Read the model definition and answer for the solid it produces. Units are mm, in the model's axes. Coordinates: 2 decimals unless noted, no trailing zeros. Write each loop counter-clockwise with the first axis right and the second up, starting at its lowest first coordinate (ties: lowest second). Pieces come first, ordered by that corner, then holes.
1) Find the intervals of material crossed by line 1 (Y direction, x = 0, z = 5.5); line 2 (Y direction, x = -15, z = 4.5); line 3 (Y direction, x = 14.5, z = 4.75), in increasing order.
2) Each of these flat-tipped pins is pushed along its axis until it touches: pin 1 Ø9 at (x, y) = (0, 64) entering from +Z; pin 2 Ø5 at (x, y) = (-36.5, 62.5) entering from -Z; pin 3 Ø3 at (x, y) = (2.5, -56.5) entering from -Z; pin 4 Ø2.5 at (x, y) = (0, -12) entering from -Z. Where does it stop, or does it pass through?
3) The part is cut by section A-A (y = -26.28). Determine the outline of the cut face in (x, z).
4) The part is cut by section D-D (y = 64). Determine the outline of the cut face in (x, z), then the cut area to 3 significant figures.
5) The part is cut by section B-B (z = 2). Give the number of separate pieces and of enclosed holes in the cut face, then the cut area to 3 significant figures.
6) The part is cut by section C-C (x = 0). Determine the outline of the cut face in (y, z), then the cut area to 3 significant figures.
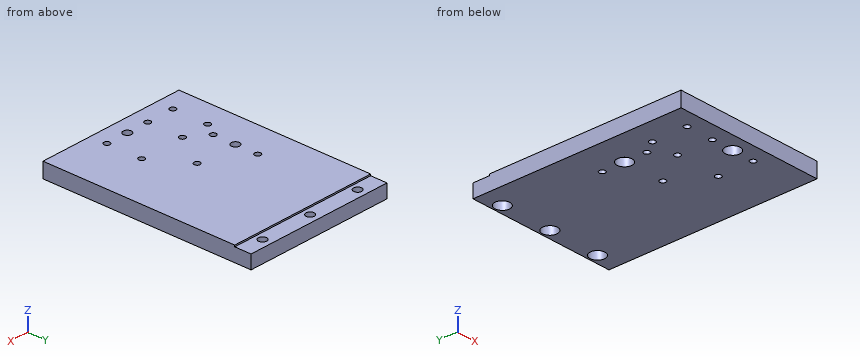
from build123d import *

# Parameters (mm, degrees)
SKIZZE1_W                                            = 100
SKIZZE1_H                                            = 140
AUFSATZ_LINEAR_AUSTRAGEN1_DEPTH                      = 10
STIRNSENKUNG_F_R_M5_ZYLINDERSCHRAUBE_MIT_D           = 5.5
STIRNSENKUNG_F_R_M5_ZYLINDERSCHRAUBE_MIT_CBORE_D     = 10
STIRNSENKUNG_F_R_M5_ZYLINDERSCHRAUBE_MIT_CBORE_DEPTH = 5.4
SKIZZE8_W                                            = 100
SKIZZE8_H                                            = 11
SCHNITT_LINEAR_AUSTRAGEN1_DEPTH                      = 1
STIRNSENKUNG_F_R_M5_ZYLINDERSCHRAUBE_2_D             = 5.5
STIRNSENKUNG_F_R_M5_ZYLINDERSCHRAUBE_2_CBORE_D       = 10
STIRNSENKUNG_F_R_M5_ZYLINDERSCHRAUBE_2_CBORE_DEPTH   = 5.4
F_4_0_4_DURCHMESSER_BOHRUNG1_D                       = 4
F_4_0_4_DURCHMESSER_BOHRUNG2_D                       = 4
F_4_0_4_DURCHMESSER_BOHRUNG3_D                       = 4
F_4_0_4_DURCHMESSER_BOHRUNG4_D                       = 4


with BuildPart() as part:
    # Skizze1 → Aufsatz-Linear austragen1 (new body)
    with BuildSketch(Plane.XY):
        Rectangle(SKIZZE1_W, SKIZZE1_H)
    extrude(amount=AUFSATZ_LINEAR_AUSTRAGEN1_DEPTH)

    # Stirnsenkung f_r M5 Zylinderschraube mit (through all)
    with Locations(Plane(origin=(0, 0, 0), x_dir=(-1, 0, 0), z_dir=(0, 0, -1))):
        with Locations((0, 64), (35, 64), (-35, 64)):
            CounterBoreHole(STIRNSENKUNG_F_R_M5_ZYLINDERSCHRAUBE_MIT_D / 2, STIRNSENKUNG_F_R_M5_ZYLINDERSCHRAUBE_MIT_CBORE_D / 2, STIRNSENKUNG_F_R_M5_ZYLINDERSCHRAUBE_MIT_CBORE_DEPTH)

    # Skizze8 → Schnitt-Linear austragen1 (cut)
    with BuildSketch(Plane.XY.offset(10)):
        with Locations((0, 64.5)):
            Rectangle(SKIZZE8_W, SKIZZE8_H)
    extrude(amount=-SCHNITT_LINEAR_AUSTRAGEN1_DEPTH, mode=Mode.SUBTRACT)

    # Stirnsenkung f_r M5 Zylinderschraube 2 (through all)
    with Locations(Plane(origin=(0, 0, 0), x_dir=(-1, 0, 0), z_dir=(0, 0, -1))):
        with Locations((0, -59), (27.37, -11.28)):
            CounterBoreHole(STIRNSENKUNG_F_R_M5_ZYLINDERSCHRAUBE_2_D / 2, STIRNSENKUNG_F_R_M5_ZYLINDERSCHRAUBE_2_CBORE_D / 2, STIRNSENKUNG_F_R_M5_ZYLINDERSCHRAUBE_2_CBORE_DEPTH)

    # Ø4.0 (4) Durchmesser Bohrung1 (through all)
    with Locations(Plane(origin=(0, 0, 0), x_dir=(-1, 0, 0), z_dir=(0, 0, -1))):
        with Locations((15, -59), (-15, -59), (27.37, -26.28), (27.37, 3.72)):
            Hole(F_4_0_4_DURCHMESSER_BOHRUNG1_D / 2)

    # Ø4.0 (4) Durchmesser Bohrung2 (through all)
    with Locations(Plane(origin=(0, 0, 0), x_dir=(-1, 0, 0), z_dir=(0, 0, -1))):
        with Locations((15, -35.6), (-15, -35.6)):
            Hole(F_4_0_4_DURCHMESSER_BOHRUNG2_D / 2)

    # Ø4.0 (4) Durchmesser Bohrung3 (through all)
    with Locations(Plane.XY.offset(10)):
        with Locations((-33.5, -35.6), (-33.5, -59)):
            Hole(F_4_0_4_DURCHMESSER_BOHRUNG3_D / 2)

    # Ø4.0 (4) Durchmesser Bohrung4 (through all)
    with Locations(Plane.XY.offset(10)):
        with Locations((0, -12)):
            Hole(F_4_0_4_DURCHMESSER_BOHRUNG4_D / 2)


solid = part.part
Reported:
1. line 1: y = -70 to -61.75, -56.25 to -14, -10 to 61.25, 66.75 to 70
1. line 2: y = -70 to -61, -57 to -37.6, -33.6 to 70
1. line 3: y = -70 to -60.94, -57.06 to -37.54, -33.66 to 70
2. pin 1: stops at z = 9
2. pin 2: stops at z = 5.4
2. pin 3: stops at z = 0
2. pin 4: passes through
3. outline: (-50, 0) - (-29.37, 0) - (-29.37, 10) - (-50, 10) - close; (-25.37, 0) - (50, 0) - (50, 10) - (-25.37, 10) - close
4. outline: (-50, 0) - (-40, 0) - (-40, 5.4) - (-37.75, 5.4) - (-37.75, 9) - (-50, 9) - close; (-32.25, 5.4) - (-30, 5.4) - (-30, 0) - (-5, 0) - (-5, 5.4) - (-2.75, 5.4) - (-2.75, 9) - (-32.25, 9) - close; (2.75, 5.4) - (5, 5.4) - (5, 0) - (30, 0) - (30, 5.4) - (32.25, 5.4) - (32.25, 9) - (2.75, 9) - close; (37.75, 5.4) - (40, 5.4) - (40, 0) - (50, 0) - (50, 9) - (37.75, 9) - close
4. area: 679 mm2
5. separate pieces: 1
5. enclosed holes: 14
5. area: 13,500 mm2
6. outline: (-70, 0) - (-64, 0) - (-64, 5.4) - (-61.75, 5.4) - (-61.75, 10) - (-70, 10) - close; (-56.25, 5.4) - (-54, 5.4) - (-54, 0) - (-14, 0) - (-14, 10) - (-56.25, 10) - close; (-10, 0) - (59, 0) - (59, 5.4) - (61.25, 5.4) - (61.25, 9) - (59, 9) - (59, 10) - (-10, 10) - close; (66.75, 5.4) - (69, 5.4) - (69, 0) - (70, 0) - (70, 9) - (66.75, 9) - close
6. area: 1,200 mm2
